from build123d import *

# Parameters (mm, degrees)
SKETCH1_W           = 45
SKETCH1_H           = 20
SKETCH1_R           = 1
BOSS_EXTRUDE1_DEPTH = 1.5
SKETCH2_R           = 8
BOSS_EXTRUDE2_DEPTH = 12
FILLET1_R           = 1


with BuildPart() as part:
    # Sketch1 → Boss-Extrude1 (new body)
    with BuildSketch(Plane(origin=(0, 0, 0), x_dir=(1, 0, 0), z_dir=(0, 1, 0))):
        with Locations((22.5, 10)):
            Rectangle(SKETCH1_W, SKETCH1_H)
        with Locations((2, 18.25)):
            Circle(SKETCH1_R, mode=Mode.SUBTRACT)
        with Locations((2, 1.75)):
            Circle(SKETCH1_R, mode=Mode.SUBTRACT)
        with Locations((43, 1.75)):
            Circle(SKETCH1_R, mode=Mode.SUBTRACT)
        with Locations((43, 18.25)):
            Circle(SKETCH1_R, mode=Mode.SUBTRACT)
    extrude(amount=BOSS_EXTRUDE1_DEPTH)

    # Sketch2 → Boss-Extrude2 (add)
    with BuildSketch(Plane(origin=(0, 1.5, 0), x_dir=(1, 0, 0), z_dir=(0, 1, 0))):
        with Locations((9.5, 10)):
            Circle(SKETCH2_R)
        with Locations((35.5, 10)):
            Circle(SKETCH2_R)
    extrude(amount=BOSS_EXTRUDE2_DEPTH)

    # Fillet1
    fillet1_edges = [part.edges().sort_by_distance(p)[0] for p in [
        (1.5, 13.5, -10),
        (27.5, 13.5, -10),
    ]]
    fillet(fillet1_edges, radius=FILLET1_R)


solid = part.part
Design review of the part built by this model. Coordinates are the model's own, in mm. A direction names the side the tool comes from. Round coordinates to 2 decimals unless told otherwise and drop trailing zeros. Order: outer loops, then holes, each group sorted by start corner. A loop starts at its lowest first (then second) coordinate and runs counter-clockwise, first axis right, second up. Notation, with made-up numbers: M 32.5,9.25 L 46.5,9.25 A17 cw 46.5,21.25 Z; hole C 80,-36.75 d9. An arc over 180 degrees is marked long. Answer as CSV lines item,"result". Start each with the question number.
1) Add section D-D (x = 43). Give the number of separate pieces and of enclosed holes in the cut face, then the cut area to 3 significant figures.
2) Add section B-B (z = -10). Give the boundary of the cut face in (x, y), then the cut area to 3 significant figures.
3) Add section A-A (x = 9.5). Give the boundary of the cut face in (y, z), then the cut area to 3 significant figures.
4) Tool access review of faces 1 (the face through (22, 1.5, -10)), 2 (the face through (43.46, 0.74, -17.36)): name each direction out of +Z, -Z, +X, -X, +Y, -Y from which nothing blocks a thin tool from reaching the whole face with its end or side.
5) For pin 1 Ø8 at (x, y) = (19.5, 6.5) entering from +Z; pin 2 Ø3 at (x, z) = (2, -1.75) entering from +Y; pin 3 Ø8 at (x, y) = (34.5, 7) entering from +Z, all flat-tipped, find the tip position at first contact; note any pin that passes through.
6) Wall thickness on line 1 along X through (y, z) = (1.2, -18.25); line 2 along Z through (x, y) = (43, 0.5); line 3 along X through (y, z) = (12, -10): over which ranges is each line inside the solid? List them lowest first. Write a range as [from, to].
7) The part is to be moulded in two halves that separate along Z. For faces 3 (the face through (29.151, 6.923, -5.132)), 4 (the face through (43.954, 0.74, -2.05)), 5 (the face through (22, 0, -10)), say which applies: +Z half, -Z half, draft (parallel to the pull), parting line (faces both ways), or undercut.
8) Add section C-C (y = 5.5). Give the boundary of the cut face in (x, z).
Resolved:
1,separate pieces,"3"
1,enclosed holes,"0"
1,area,"89.2 mm^2"
2,outline,"M 0,0 L 45,0 L 45,1.5 L 43.5,1.5 L 43.5,12.5 A1 ccw 42.5,13.5 L 28.5,13.5 A1 ccw 27.5,12.5 L 27.5,1.5 L 17.5,1.5 L 17.5,12.5 A1 ccw 16.5,13.5 L 2.5,13.5 A1 ccw 1.5,12.5 L 1.5,1.5 L 0,1.5 Z"
2,area,"451 mm^2"
3,outline,"M 0,-20 L 1.5,-20 L 1.5,-18 L 12.5,-18 A1 ccw 13.5,-17 L 13.5,-3 A1 ccw 12.5,-2 L 1.5,-2 L 1.5,0 L 0,0 Z"
3,area,"222 mm^2"
4,face 1,"+Y"
4,face 2,"+Y, -Y"
5,pin 1,"z = -4.71"
5,pin 2,"y = 1.5"
5,pin 3,"z = -2"
6,line 1,"[0, 1], [3, 42], [44, 45]"
6,line 2,"[-20, -19.25], [-17.25, -2.75], [-0.75, 0]"
6,line 3,"[1.5, 17.5], [27.5, 43.5]"
7,face 3,"parting line"
7,face 4,"undercut"
7,face 5,"draft"
8,outline,"C 9.5,-10 d16; C 35.5,-10 d16"
